Model file for the job. Use its own axes, mm. A direction names the side the tool comes from. Round coordinates to 2 decimals unless told otherwise and drop trailing zeros. Write each loop counter-clockwise with the first axis right and the second up, starting at its lowest first coordinate (ties: lowest second). Pieces come first, ordered by that corner, then holes. Notation, with made-up numbers: (5.25, 58) - (11.25, 58) arc R21 cw to (11.25, 73) - close; hole circle Ø5 at (70, 24.25). An arc over 180 degrees is marked (long way). One line per item, written item: value.
Autodesk Fusion 360 part; units mm, degrees
sketch "Sketch1" plane through (0, 0, 0) normal (0, 0, 1) x (1, 0, 0)
  circle A0 centre (0, 0) radius 3.7
  circle A1 centre (0, 0) radius 6
  line L0 (-25, -13.2) -> (25, -13.2)
  line L1 (25, -13.2) -> (25, -17.2)
  line L2 (25, -17.2) -> (-25, -17.2)
  line L3 (-25, -17.2) -> (-25, -13.2)
  line L4 (-6, 0) -> (6, 0)
  line L5 (6, 0) -> (6, -13.2)
  line L6 (6, -13.2) -> (-6, -13.2)
  line L7 (-6, -13.2) -> (-6, 0)
  point P0 (0, -13.2)
  dimension "d1" = 7.4
  dimension "d2" = 12
  dimension "d7" = 50
  dimension "d8" = 13.2
  dimension "d30" = 4
extrude "Extrude1" add sketch "Sketch1" along normal blind 2 contours A0 L4 | A0 A1 L4 | A0 A1 L4 | A0 L4
extrude "Extrude2" add sketch "Sketch1" along normal blind 18 contours A0 A1 L4 | A0 A1 L4
extrude "Extrude3" add sketch "Sketch1" along normal blind 12 contours A1 L0 L5 L6 L7
extrude "Extrude4" add sketch "Sketch1" along normal blind 30 contours L0 L1 L2 L3 L6
sketch "Sketch4" plane through (0, -13.2, 0) normal (0, 1, 0) x (-1, 0, 0)
  line L0 (6, 12) -> (6, 0)
  line L1 (6, 0) -> (25, 0)
  line L2 (25, 0) -> (25, 30)
  line L3 (25, 30) -> (-25, 30)
  line L4 (-25, 30) -> (-25, 0)
  line L5 (-25, 0) -> (-6, 0)
  line L6 (-6, 0) -> (-6, 12)
  line L7 (-6, 12) -> (6, 12)
  circle A0 centre (-19, 15) radius 1.5
  circle A1 centre (19, 15) radius 1.5
  point P0 (-25, 15)
  point P1 (25, 15)
  dimension "d31" = 3
  dimension "d32" = 3
  dimension "d33" = 6
  dimension "d35" = 6
chamfer "Chamfer1" distance 2 distance2 30 1 edges at (0, -17.2, 0) measured on face at (-2, -4.4, 0)
extrude "Extrude8" cut sketch "Sketch4" against normal blind 16 contours A0 | A1
1. Mould opens along X. For faces 4 (the face through (-3, -3, 18)), 5 (the face through (-25, -15, 15)), 6 (the face through (0, 0, 2)), 7 (the face through (-18.805, -14.729, 16.487)) say: released by +X, released by -X, zero draft, split by the parting line, or undercut.
Report:
face 4: zero draft
face 5: released by -X
face 6: undercut
face 7: undercut
2. Wall check: probe 1 along X at (y, z) = (-15.45, 15); probe 2 along Z at (x, y) = (-19, -14.55); probe 3 along X at (y, z) = (0, 8). Give the ranges that are in metal, low to high. Write a range as [from, to].
Report:
probe 1: [-25, -20.5], [-17.5, 17.5], [20.5, 25]
probe 2: [0, 13.5], [16.5, 30]
probe 3: [-6, -3.7], [3.7, 6]
3. Band-saw the part on C-C on y = -1.75. Write the cut outline in (x, z).
Report:
outline: (-6, 0) - (6, 0) - (6, 12) - (5.74, 12) - (5.74, 18) - (3.26, 18) - (3.26, 2) - (-3.26, 2) - (-3.26, 18) - (-5.74, 18) - (-5.74, 12) - (-6, 12) - close
4. Tool access for faces 1 (the face through (-0.802, 3.612, 9.888)), 2 (the face through (6, -7, 6)), 3 (the face through (-6, -7, 6)): list every direction of +Z, -Z, +X, -X, +Y, -Y with a clear straight run to the whole face (end or side of a thin tool).
Report:
face 1: +Z
face 2: +Z, -Z, +X, +Y
face 3: +Z, -Z, -X, +Y
5. Drop flat-ended pins along their axis: pin 1 (3.5 mm diameter, centred on x = -1, y = -0.5, fed in from +Z); pin 2 (3.5 mm diameter, centred on y = -6, z = 6.5, fed in from +X); pin 3 (8.5 mm diameter, centred on x = 0, y = 0, fed in from +Z). Give the stop position or say it passes through.
Report:
pin 1: z = 2
pin 2: x = 6
pin 3: z = 18
6. Band-saw the part on B-B on z = 15. Write the cut outline in (x, y), plus the area to 3 significant figures.
Report:
outline: (-25, -16.2) - (-20.5, -16.2) - (-20.5, -13.2) - (-25, -13.2) - close; (-17.5, -16.2) - (17.5, -16.2) - (17.5, -13.2) - (-17.5, -13.2) - close; circle Ø12 at (0, 0); (20.5, -16.2) - (25, -16.2) - (25, -13.2) - (20.5, -13.2) - close; hole circle Ø7.4 at (0, 0)
area: 202 mm²
